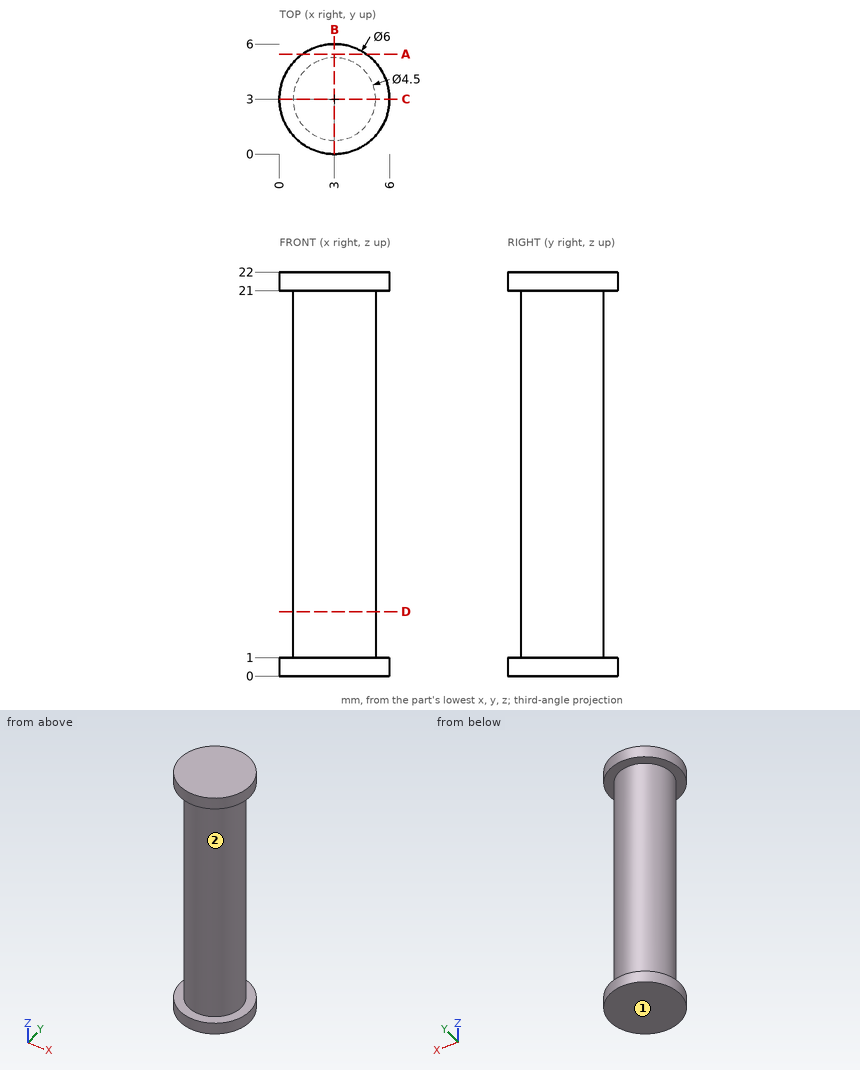
Study the drawing (mm; zero at the part's minimum x, y, z) and answer. A direction names the side the tool comes from. Round coordinates to 2 decimals unless told otherwise and drop trailing zeros. Order: outer loops, then holes, each group sorted by start corner. A loop starts at its lowest first (then second) coordinate and runs counter-clockwise, first axis right, second up. Notation, with made-up numbers: (-31, -11.5) - (-19, -11.5) arc R18 cw to (-19, 20.5) - close; hole circle Ø10 at (46, 15.25). An arc over 180 degrees is marked (long way). Use one line per item in the form item = value. Start each with the question number.
(1) Find the intervals of material crossed by line 1 along Z through (x, y) = (4.7, 0.6); line 2 along Y through (x, z) = (2.95, 6); line 3 along Y through (x, z) = (4.15, 3.75), in increasing order. Write a range as from..to.
(2) For the marked faces 1 and 2, determine the directions among +Z, -Z, +X, -X, +Y, -Y from which every point of the face is accessible in a straight line to the end or side of a thin tool.
(3) The part is cut by section A-A (y = 5.45). Give the vertices of the cut face in (x, z).
(4) The part is cut by section B-B (x = 3). Give the vertices of the cut face in (y, z), then the cut area to 3 significant figures.
(5) A flat-ended cylindrical pin translates along its axis: pin 1 Ø3 at (x, z) = (4, 10.5) entering from -Y. Find the tip coordinate at first contact, or state that the pin passes through.
(6) The part is cut by section D-D (z = 3.5). Give the vertices of the cut face in (x, y), then the cut area to 3 significant figures.
Checked values:
q1.line_1 = 0..1, 21..22
q1.line_2 = 0.75..5.25
q1.line_3 = 1.07..4.93
q2.face_1 = -Z, +X, -X, +Y, -Y
q2.face_2 = none
q3.outline = (1.27, 0) - (4.73, 0) - (4.73, 1) - (1.27, 1) - close; (1.27, 21) - (4.73, 21) - (4.73, 22) - (1.27, 22) - close
q4.outline = (0, 0) - (6, 0) - (6, 1) - (5.25, 1) - (5.25, 21) - (6, 21) - (6, 22) - (0, 22) - (0, 21) - (0.75, 21) - (0.75, 1) - (0, 1) - close
q4.area = 102 mm^2
q5.pin_1 = 0.75
q6.outline = circle Ø4.5 at (3, 3)
q6.area = 15.9 mm^2
